Verification items for the finished model (mm, model axes). A direction names the side the tool comes from. Round coordinates to 2 decimals unless told otherwise and drop trailing zeros. Write each loop counter-clockwise with the first axis right and the second up, starting at its lowest first coordinate (ties: lowest second). Pieces come first, ordered by that corner, then holes. Notation, with made-up numbers: (30, 53) -> (85, 53) arc R17 ccw to (85, 70) -> close; hole circle Ø4 at (64, 31.25). An arc over 180 degrees is marked (long way). Answer as a JSON object with one key per item and string values. Group by question number.
(1) Gauge pin test, flat ends, axial feed: pin 1 Ø1.2 at (y, z) = (-7.78, 19.22) entering from -X; pin 2 Ø1.6 at (x, z) = (0, 30) entering from +Y. Record the tip position at first contact, or that the pin passes through.
(2) Sectioned sample at C-C on y = 13.5. Record the cut outline in (x, z).
(3) Sectioned sample at B-B on y = 0. Record the cut outline in (x, z), and give its area (3 significant figures).
(4) Sectioned sample at A-A on z = 27. Record the cut outline in (x, y).
(5) Sectioned sample at D-D on x = 0. Count the separate pieces of the cut face and the enclosed holes in it, and give its area (3 significant figures).
(6) Set-up check for faces 1 (the face through (-2, 0, 40)), 2 (the face through (0, 18, 31)): record each of +Z, -Z, +X, -X, +Y, -Y from which the full face is reachable in a straight line by a thin tool's end or side.
(7) Draft check along Y on faces 3 (the face through (0, -25, 1)), 4 (the face through (-5, 6, 1)), 5 (the face through (1, 25, 1)), 6 (the face through (0.07, 8.32, -18.38)). Enter one of: released by +Y, released by -Y, zero draft, split by the parting line, or undercut.
(8) Scan lines: L1, parallel to Y at x = -2.5, z = 34.5; L2, parallel to Y at x = -1.5, z = -35.5; L3, parallel to Z at x = -1.5, y = 0. Record each from-to range of solid material in increasing order. Write a range as from..to.
Solid Edge part; units mm, degrees
sketch "Sketch1" plane through (0, 0, 0) normal (0, -1, 0) x (1, 0, 0)
  line L0 (-5, -40) -> (5, -40)
  line L1 (5, -40) -> (5, 40)
  line L2 (5, 40) -> (-5, 40)
  line L3 (-5, 40) -> (-5, -40)
  dimension "D1" = 5
  dimension "D2" = 5
extrude "Protrusion1" add sketch "Sketch1" along normal mid plane 50
sketch "Sketch2" plane through (5, 0, 0) normal (1, 0, 0) x (0, 1, 0)
  circle A0 centre (0, 0) radius 4.4
extrude "Cutout1" cut sketch "Sketch2" against normal through all
sketch "Sketch3" plane through (5, 0, 0) normal (1, 0, 0) x (0, 1, 0)
  circle A0 centre (-7.7782, 34.7782) radius 1
  circle A1 centre (-7.7782, 19.2218) radius 1
  circle A2 centre (7.7782, 19.2218) radius 1
  circle A3 centre (7.7782, 34.7782) radius 1
  circle A4 centre (0, 27) radius 5
  dimension "D1" = 7.7782
extrude "Cutout2" cut sketch "Sketch3" against normal through all
mirror "Mirror1" about plane through (0, 0, 0) normal (0, 0, 1) of "Cutout2"
sketch "Sketch4" plane through (0, 25, 0) normal (0, 1, 0) x (-1, 0, 0)
  circle A0 centre (0, 30) radius 1
  circle A1 centre (0, 0) radius 1
  circle A2 centre (0, -30) radius 1
  dimension "D1" = 0.0001
extrude "Extrusionsausschnitt_6" cut sketch "Sketch4" against normal blind 15
fillet "Verrundung_3" radius 4 2 edges at (5, 0, 40) (5, 0, -40)
properties material "Nylon, allgemein"
Computed values:
{
 "1": {"pin 1": "through", "pin 2": "y = 10"},
 "2": {"outline": "(-5, -40) -> (1, -40) arc R4 ccw to (5, -36) -> (5, 36) arc R4 ccw to (1, 40) -> (-5, 40) -> close; hole circle Ø2 at (0, -30); hole circle Ø2 at (0, 0); hole circle Ø2 at (0, 30)"},
 "3": {"outline": "(-5, -40) -> (1, -40) arc R4 ccw to (5, -36) -> (5, -32) -> (-5, -32) -> close; (-5, -22) -> (5, -22) -> (5, -4.4) -> (-5, -4.4) -> close; (-5, 4.4) -> (5, 4.4) -> (5, 22) -> (-5, 22) -> close; (-5, 32) -> (5, 32) -> (5, 36) arc R4 ccw to (1, 40) -> (-5, 40) -> close", "area": "505 mm2"},
 "4": {"outline": "(-5, -25) -> (5, -25) -> (5, -5) -> (-5, -5) -> close; (-5, 5) -> (5, 5) -> (5, 25) -> (-5, 25) -> close"},
 "5": {"separate pieces": "1", "enclosed holes": "11", "area": "3,670 mm2"},
 "6": {"face 1": "+Z, +X, -X, +Y, -Y", "face 2": "+Y"},
 "7": {"face 3": "released by -Y", "face 4": "zero draft", "face 5": "released by +Y", "face 6": "undercut"},
 "8": {"L1": "-25..-8.74, -6.82..6.82, 8.74..25", "L2": "-25..-8.47, -7.09..7.09, 8.47..25", "L3": "-40..-32, -22..-4.4, 4.4..22, 32..40"}
}
